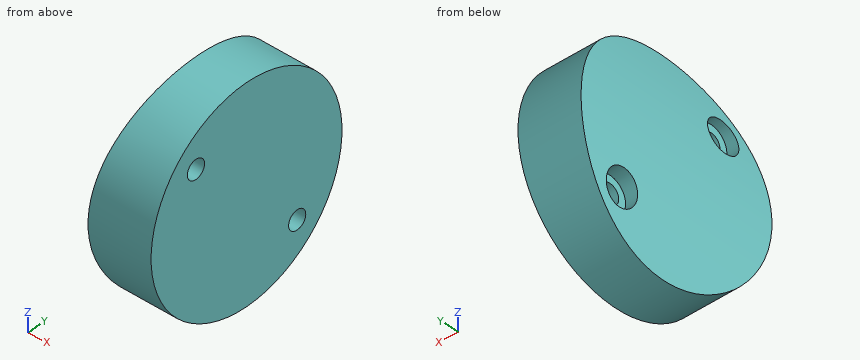
```python
from build123d import *

# Parameters (mm, degrees)
SKETCH1_R                              = 20
BLOCO_DEPTH                            = 12
FURO_DE_FIXA_O_PARAFUSO_M3_D           = 3.6
FURO_DE_FIXA_O_PARAFUSO_M3_CBORE_D     = 6.5
FURO_DE_FIXA_O_PARAFUSO_M3_CBORE_DEPTH = 3
CORTE_ARREDONDAMENTO_DEPTH             = 31.724582991
CORTE_ARREDONDAMENTO_DEPTH_BACK        = 31.724582991
SKETCH7_R                              = 100
SKETCH7_R_2                            = 75


with BuildPart() as part:
    # Sketch1 → Bloco (new body)
    with BuildSketch(Plane(origin=(0, 0, 0), x_dir=(0, 0, -1), z_dir=(1, 0, 0))):
        Circle(SKETCH1_R)
    extrude(amount=BLOCO_DEPTH)

    # Furo de Fixação - Parafuso M3 (through all)
    with Locations(Plane.ZY):
        with Locations((10.606601718, -10.606601718), (-10.606601718, 10.606601718)):
            CounterBoreHole(FURO_DE_FIXA_O_PARAFUSO_M3_D / 2, FURO_DE_FIXA_O_PARAFUSO_M3_CBORE_D / 2, FURO_DE_FIXA_O_PARAFUSO_M3_CBORE_DEPTH)

    # Sketch7 → Corte - Arredondamento (cut, two sides: drawn at the far end of the back side and taken through both)
    with BuildSketch(Plane(origin=(0, 0, 0), x_dir=(1, 0, 0), z_dir=(0, 1, 0)).offset(-CORTE_ARREDONDAMENTO_DEPTH_BACK)):
        with Locations((75, 0)):
            Circle(SKETCH7_R)
        with Locations((75, 0)):
            Circle(SKETCH7_R_2, mode=Mode.SUBTRACT)
    extrude(amount=CORTE_ARREDONDAMENTO_DEPTH + CORTE_ARREDONDAMENTO_DEPTH_BACK, mode=Mode.SUBTRACT)


solid = part.part
```
Input: part model. Units: mm. Frame: model coordinates. Give positions to 0.01 mm unless a question says otherwise; leave off trailing zeros. Order: outer loops, then holes, each group sorted by start corner. A loop starts at its lowest first (then second) coordinate and runs counter-clockwise, first axis right, second up. Notation, with made-up numbers: (-36.75, 74.5) - (-23.75, 74.5) arc R35 cw to (-23.75, 110.5) - close; hole circle Ø8 at (-3.5, 25). An arc over 180 degrees is marked (long way). Put each result on its own line as item: value.
Item 1: Section query B-B, the plane z = 3. Return loops of the section in (x, y), then the cut area to 3 significant figures.
Found:
outline: (0.06, -19.77) - (12, -19.77) - (12, 19.77) - (0.06, 19.77) - close
area: 472 mm^2
Item 2: Section query C-C, the plane x = 8. Return loops of the section in (y, z).
Found:
outline: circle Ø40 at (0, 0); hole circle Ø3.6 at (-10.61, 10.61); hole circle Ø3.6 at (10.61, -10.61)
Item 3: Ray query, L1, parallel to Z at x = 2.5, y = 11; L2, parallel to Y at x = 5.75, z = 12; L3, parallel to Y at x = 3.75, z = 0. Return the intervals inside material, ascending. Write a range as from..to.
Found:
L1: z = -16.7..-13.83, -7.38..16.7
L2: y = -16..-11.75, -9.47..16
L3: y = -20..20
Item 4: Contact query for flat-ended pins moving along their axis: pin 1 (5 mm diameter, centred on y = 10.5, z = -11.5, fed in from -X); pin 2 (6 mm diameter, centred on x = 9, z = -14.5, fed in from +Y); pin 3 (2 mm diameter, centred on y = -10, z = 3, fed in from -X). Output: stop coordinate, or through.
Found:
pin 1: stops at x = 1.18
pin 2: stops at y = 16.36
pin 3: stops at x = 0.03
Item 5: Section query A-A, the plane y = 0. Return loops of the section in (x, z), then the cut area to 3 significant figures.
Found:
outline: (2.72, -20) - (12, -20) - (12, 20) - (2.72, 20) arc R75 ccw to start
area: 444 mm^2
